Geometry check sheet. Reference: the model listing, model coordinates, mm. Face numbers are marked on the shaded views. A direction names the side the tool comes from. Give positions to 0.01 mm unless a question says otherwise; leave off trailing zeros. Order: outer loops, then holes, each group sorted by start corner. A loop starts at its lowest first (then second) coordinate and runs counter-clockwise, first axis right, second up. Notation, with made-up numbers: M -22.5,-40 L 32.5,-40 A12 ccw 32.5,-25 Z; hole C -4.5,-40 d7. An arc over 180 degrees is marked long. Answer as CSV lines item,"result".
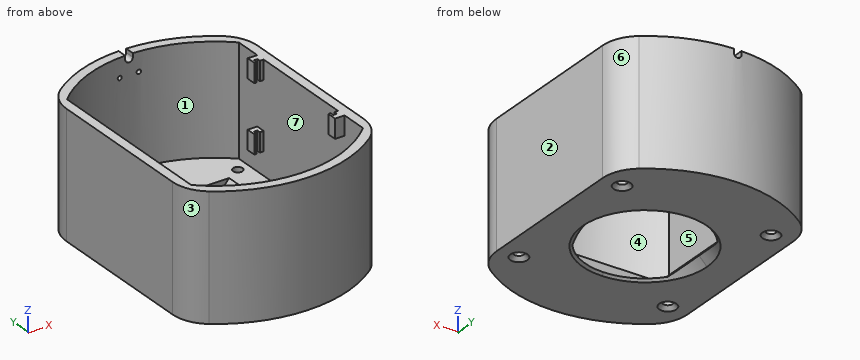
from build123d import *

# Parameters (mm, degrees)
EXTRUDE_2_DEPTH     = 65
SKETCH_1_3_R        = 2.5
BOSS_EXTRUDE1_DEPTH = 8
FILLET1_R           = 20
CHAMFER3_SIZE       = 5
BOSS_EXTRUDE3_DEPTH = 10
BOSS_EXTRUDE4_START = -45
BOSS_EXTRUDE4_DEPTH = 10
CUT_EXTRUDE2_DEPTH  = 108.819293264
SKETCH5_4_R         = 1.1
CUT_EXTRUDE3_DEPTH  = 68
CUT_EXTRUDE4_DEPTH  = 35
CHAMFER4_SIZE       = 2


with BuildPart() as part:
    # Sketch 1 → Extrude 2 (new body)
    with BuildSketch(Plane.XY):
        with BuildLine():
            Line((-50, -48.989794856), (-50, 48.989794856))
            ThreePointArc((-50, 48.989794856), (0, 70), (50, 48.989794856))
            Line((50, 48.989794856), (50, -48.989794856))
            ThreePointArc((50, -48.989794856), (0, -70), (-50, -48.989794856))
        make_face()
        with BuildLine():
            ThreePointArc((45, 46.904157598), (0, 65), (-45, 46.904157598))
            Line((-45, 46.904157598), (-45, -46.904157598))
            ThreePointArc((-45, -46.904157598), (0, -65), (45, -46.904157598))
            Line((45, -46.904157598), (45, 46.904157598))
        make_face(mode=Mode.SUBTRACT)
    extrude(amount=EXTRUDE_2_DEPTH)

    # Sketch 1_3 → Boss-Extrude1 (add)
    with BuildSketch(Plane.XY):
        with BuildLine():
            Line((45, -46.904157598), (45, 46.904157598))
            ThreePointArc((45, 46.904157598), (0, 65), (-45, 46.904157598))
            Line((-45, 46.904157598), (-45, -46.904157598))
            ThreePointArc((-45, -46.904157598), (0, -65), (45, -46.904157598))
        make_face()
        with Locations((39, -39)):
            Circle(SKETCH_1_3_R, mode=Mode.SUBTRACT)
        with BuildLine():
            Line((27.5, 0.1), (27.5, -0.1))
            ThreePointArc((27.5, -0.1), (19.474725805, -19.474725805), (0.1, -27.5))
            Line((0.1, -27.5), (-0.1, -27.5))
            ThreePointArc((-0.1, -27.5), (-19.474725805, -19.474725805), (-27.5, -0.1))
            Line((-27.5, -0.1), (-27.5, 0.1))
            ThreePointArc((-27.5, 0.1), (-19.474725805, 19.474725805), (-0.1, 27.5))
            Line((-0.1, 27.5), (0.1, 27.5))
            ThreePointArc((0.1, 27.5), (19.474725805, 19.474725805), (27.5, 0.1))
        make_face(mode=Mode.SUBTRACT)
        with Locations((39, 39)):
            Circle(SKETCH_1_3_R, mode=Mode.SUBTRACT)
        with Locations((-39, -39)):
            Circle(SKETCH_1_3_R, mode=Mode.SUBTRACT)
        with Locations((-39, 39)):
            Circle(SKETCH_1_3_R, mode=Mode.SUBTRACT)
    extrude(amount=BOSS_EXTRUDE1_DEPTH)

    # Fillet1
    fillet1_edges = [part.edges().sort_by_distance(p)[0] for p in [
        (-50, 48.989794856, 32.5),
        (50, 48.989794856, 32.5),
        (50, -48.989794856, 32.5),
        (-50, -48.989794856, 32.5),
    ]]
    fillet(fillet1_edges, radius=FILLET1_R)

    # Chamfer3
    chamfer3_edges = [part.edges().sort_by_distance(p)[0] for p in [
        (0, 27.5, 0),
        (19.474725805, 19.474725805, 0),
        (27.5, 0, 0),
        (19.474725805, -19.474725805, 0),
        (-19.474725805, 19.474725805, 0),
        (-27.5, 0, 0),
        (-19.474725805, -19.474725805, 0),
        (0, -27.5, 0),
    ]]
    chamfer(chamfer3_edges, length=CHAMFER3_SIZE)

    # Sketch3 → Boss-Extrude3 (add)
    with BuildSketch(Plane.XY.offset(65)):
        Polygon((41.2, -30), (41.2, -28), (40, -28), (40, -33), (45, -33), (45, -28.104490543), (43, -28.104490543), (43, -30), align=None)
        Polygon((45, 28.104490543), (45, 33), (40, 33), (40, 28), (41.2, 28), (41.2, 30), (43, 30), (43, 28.104490543), align=None)
    extrude(amount=-BOSS_EXTRUDE3_DEPTH)

    # Sketch3_2 → Boss-Extrude4 (add)
    with BuildSketch(Plane.XY.offset(65).offset(BOSS_EXTRUDE4_START)):
        Polygon((41.2, -30), (41.2, -28), (40, -28), (40, -33), (45, -33), (45, -28.104490543), (43, -28.104490543), (43, -30), align=None)
        Polygon((45, 28.104490543), (45, 33), (40, 33), (40, 28), (41.2, 28), (41.2, 30), (43, 30), (43, 28.104490543), align=None)
    extrude(amount=BOSS_EXTRUDE4_DEPTH)

    # Sketch5 → Cut-Extrude2 (cut, through all)
    with BuildSketch(Plane(origin=(0, 0, 0), x_dir=(1, 0, 0), z_dir=(0, 1, 0))):
        with BuildLine():
            ThreePointArc((2, -63), (1.414213562, -61.585786438), (0, -61))
            Line((0, -61), (0, -65))
            Line((0, -65), (2, -65))
            Line((2, -65), (2, -63))
        make_face()
        with BuildLine():
            Line((0, -65), (0, -61))
            ThreePointArc((0, -61), (-1.414213562, -61.585786438), (-2, -63))
            Line((-2, -63), (-2, -65))
            Line((-2, -65), (0, -65))
        make_face()
    extrude(amount=CUT_EXTRUDE2_DEPTH, mode=Mode.SUBTRACT)

    # Sketch5_4 → Cut-Extrude3 (cut)
    with BuildSketch(Plane(origin=(0, 0, 0), x_dir=(1, 0, 0), z_dir=(0, 1, 0))):
        with Locations(Location((5, -55, 0), (0, 0, 90))):
            Circle(SKETCH5_4_R)
        with Locations(Location((-5, -55, 0), (0, 0, 90))):
            Circle(SKETCH5_4_R)
    extrude(amount=CUT_EXTRUDE3_DEPTH, mode=Mode.SUBTRACT)

    # Sketch6 → Cut-Extrude4 (cut, symmetric)
    with BuildSketch(Plane(origin=(0, 0, 0), x_dir=(1, 0, 0), z_dir=(0, 1, 0))):
        with BuildLine():
            Line((25, -1.25), (0, -1.25))
            Line((0, -1.25), (0, -8))
            Line((0, -8), (0.1, -8))
            Line((0.1, -8), (31.643522244, -8))
            ThreePointArc((31.643522244, -8), (28.522145397, -4.427776683), (25, -1.25))
        make_face()
        with BuildLine():
            Line((0, -8), (0, -1.25))
            Line((0, -1.25), (-25, -1.25))
            ThreePointArc((-25, -1.25), (-28.522145397, -4.427776683), (-31.643522244, -8))
            Line((-31.643522244, -8), (-0.1, -8))
            Line((-0.1, -8), (0, -8))
        make_face()
    extrude(amount=CUT_EXTRUDE4_DEPTH, both=True, mode=Mode.SUBTRACT)

    # Chamfer4
    chamfer4_edges = [part.edges().sort_by_distance(p)[0] for p in [
        (36.5, -39, 0),
        (-41.5, 39, 0),
        (-41.5, -39, 0),
        (36.5, 39, 0),
    ]]
    chamfer(chamfer4_edges, length=CHAMFER4_SIZE)


solid = part.part
(1) Draft check along Y on the marked faces 1, 2, 3 and 4. Enter one of: +Y half, -Y half, draft (parallel to the pull), parting line (faces both ways), or undercut.
The answers:
face 1,"undercut"
face 2,"draft"
face 3,"-Y half"
face 4,"undercut"
(2) Tool access check on the marked faces 5, 6 and 7. Record the directions out of +Z, -Z, +X, -X, +Y, -Y that give a thin tool (end or side, any length) a straight path to the whole face; none if there is none.
The answers:
face 5,"+Z"
face 6,"+Z, -Z, +X, +Y"
face 7,"none"
(3) Gauge pin test, flat ends, axial feed: P1, Ø2, axis at y = 44, z = 10.5, coming from the -X side; P2, Ø2, axis at x = 14.5, y = -41, coming from the +Z side; P3, Ø2, axis at x = -8, z = 4.5, coming from the +Y side. Record the tip position at first contact, or that the pin passes through.
The answers:
P1,"stops at x = -49.77"
P2,"stops at z = 8"
P3,"stops at y = 69.65"
(4) Section check B-B on y = 52.5. Enter the section's corners in (x, z), then the cut area to 3 significant figures.
The answers:
outline,"M -45.61,0 L 45.61,0 L 45.61,65 L 38.32,65 L 38.32,8 L -38.32,8 L -38.32,65 L -45.61,65 Z"
area,"1,560 mm2"
(5) Material ranges on line 1 (X direction, y = 10, z = 10.5); line 2 (Y direction, x = -39, z = 3); line 3 (Z direction, x = 5, y = 66.3), recorded low to high.
The answers:
line 1,"x = -50 to -45, 45 to 50"
line 2,"y = -58.13 to -41.5, -36.5 to 36.5, 41.5 to 58.13"
line 3,"z = 0 to 53.9, 56.1 to 65"
(6) Section check A-A on z = 28. Enter the section's corners in (x, y), then the cut area to 3 significant figures.
The answers:
outline,"M -50,-40 A20 ccw -42,-56 A70 ccw 42,-56 A20 ccw 50,-40 L 50,40 A20 ccw 42,56 A70 ccw -42,56 A20 ccw -50,40 Z; hole M -45,-46.9 A65 ccw 45,-46.9 L 45,-33 L 40,-33 L 40,-28 L 41.2,-28 L 41.2,-30 L 43,-30 L 43,-28.1 L 45,-28.1 L 45,28.1 L 43,28.1 L 43,30 L 41.2,30 L 41.2,28 L 40,28 L 40,33 L 45,33 L 45,46.9 A65 ccw -45,46.9 Z"
area,"2,010 mm2"
(7) Section check C-C on x = -38.5. State how many separate pieces and enclosed holes the cut face has, then the cut area to 3 significant figures.
The answers:
separate pieces,"3"
enclosed holes,"0"
area,"1,540 mm2"
